from build123d import *

# Parameters (mm, degrees)
F0_R          = 3.175
F1_DEPTH      = 7.62
F2_R          = 4.445
F3_DEPTH      = 60.96
F4_R          = 3.175
F5_DEPTH      = 7.62
F6_R          = 1.905
F7_DEPTH      = 25.4
F7_DEPTH_BACK = 25.4
F8_R          = 1.905
F9_DEPTH      = 76.201


with BuildPart() as f1:
    # F0 (on Top) → F1 (new body)
    with BuildSketch(Plane.XY):
        Circle(F0_R)
    extrude(amount=F1_DEPTH)

    # F2 (on face) → F3 (join)
    with BuildSketch(Plane.XY.offset(7.62)):
        Circle(F2_R)
    extrude(amount=F3_DEPTH)

    # F4 (on face) → F5 (join)
    with BuildSketch(Plane.XY.offset(68.58)):
        Circle(F4_R)
    extrude(amount=F5_DEPTH)

    # F6 (on Front) → F7 (cut, two sides)
    with BuildSketch(Plane.XZ) as f7_sk:
        with Locations((0, 38.1)):
            Circle(F6_R)
    extrude(amount=-F7_DEPTH, mode=Mode.SUBTRACT)
    extrude(f7_sk.sketch, amount=F7_DEPTH_BACK, mode=Mode.SUBTRACT)

    # F8 (on face) → F9 (cut, through all)
    with BuildSketch(Plane(origin=(0, 0, 0), x_dir=(1, 0, 0), z_dir=(0, 0, -1))):
        Circle(F8_R)
    extrude(amount=-F9_DEPTH, mode=Mode.SUBTRACT)


solid = f1.part
The model under review builds one solid part; all positions refer to its coordinate system, in mm. A direction names the side the tool comes from. Round coordinates to 2 decimals unless told otherwise and drop trailing zeros. Loops run counter-clockwise (first coordinate to the right, second up) from the corner with the lowest first, then second, coordinate; pieces in that order, holes last. Notation, with made-up numbers: M -16.75,59.25 L 7.25,59.25 A31 ccw 7.25,89.25 Z; hole C -29,-14.75 d4. An arc over 180 degrees is marked long. Answer as a JSON object with one key per item and string values.
Item 1: Tool access review of faces 4 (the face through (-0.41, 1.86, 18.78)), 5 (the face through (-0.69, -3.1, 3.76)), 6 (the face through (-0.69, -3.1, 72.34)): name each direction out of +Z, -Z, +X, -X, +Y, -Y from which nothing blocks a thin tool from reaching the whole face with its end or side.
Check sheet entries:
{"face 4": "+Z, -Z", "face 5": "-Z", "face 6": "+Z"}
Item 2: We need section B-B, the plane y = -0.75. State the section outline as (x, z) points (3 decimals), and give its area (3 significant figures).
Check sheet entries:
{"outline": "M -4.381,7.62 L -3.085,7.62 L -3.085,0 L -1.751,0 L -1.751,37.35 A1.905 cw -1.751,38.85 L -1.751,76.2 L -3.085,76.2 L -3.085,68.58 L -4.381,68.58 Z; M 1.751,0 L 3.085,0 L 3.085,7.62 L 4.381,7.62 L 4.381,68.58 L 3.085,68.58 L 3.085,76.2 L 1.751,76.2 L 1.751,38.85 A1.905 cw 1.751,37.35 Z", "area": "361 mm2"}
Item 3: For line 1 along Y through (x, z) = (0, 24.5) (3 decimals); line 2 along Z through (x, y) = (0, 2.7) (3 decimals); line 3 along X through (y, z) = (1.25, 18.5), list the stretches that pass through material, from the lowest coordinate up.
Check sheet entries:
{"line 1": "-4.445 to -1.905, 1.905 to 4.445", "line 2": "0 to 36.195, 40.005 to 76.2", "line 3": "-4.27 to -1.44, 1.44 to 4.27"}
Item 4: We need section C-C, the plane z = 30. State the section outline as (x, y) points (3 decimals), and give its area (3 significant figures).
Check sheet entries:
{"outline": "C 0,0 d8.89; hole C 0,0 d3.81", "area": "50.7 mm2"}
Item 5: Clearance check with flat-ended pins moving along their axes: P1, Ø4, axis at y = 1.5, z = 8.5, coming from the -X side (3 decimals); P2, Ø1.5, axis at y = -3, z = 53, coming from the +X side. State where each tip first meets the part, or that it passes through.
Check sheet entries:
{"P1": "x = -4.445", "P2": "x = 3.83"}
Item 6: The part is to be moulded in two halves that separate along Y. For faces 1 (the face through (1.76, 0.73, 56.88)), 2 (the face through (4.24, 1.34, 37.67)), 3 (the face through (2, -3, 7.62)), say which applies: +Y half, -Y half, draft (parallel to the pull), parting line (faces both ways), or undercut.
Check sheet entries:
{"face 1": "undercut", "face 2": "parting line", "face 3": "draft"}
Item 7: We need section A-A, the plane x = 0. State the section outline as (y, z) points (3 decimals).
Check sheet entries:
{"outline": "M -4.445,7.62 L -3.175,7.62 L -3.175,0 L -1.905,0 L -1.905,36.195 L -4.445,36.195 Z; M -4.445,40.005 L -1.905,40.005 L -1.905,76.2 L -3.175,76.2 L -3.175,68.58 L -4.445,68.58 Z; M 1.905,0 L 3.175,0 L 3.175,7.62 L 4.445,7.62 L 4.445,36.195 L 1.905,36.195 Z; M 1.905,40.005 L 4.445,40.005 L 4.445,68.58 L 3.175,68.58 L 3.175,76.2 L 1.905,76.2 Z"}
